Design review of the part built by this model. Coordinates are the model's own, in mm. A direction names the side the tool comes from. Round coordinates to 2 decimals unless told otherwise and drop trailing zeros. Loops run counter-clockwise (first coordinate to the right, second up) from the corner with the lowest first, then second, coordinate; pieces in that order, holes last. Notation, with made-up numbers: M 3,27 L 11,27 A12 ccw 11,34 Z; hole C -32.5,89.5 d10. An arc over 180 degrees is marked long. One line per item, written item: value. Start each with the question number.
Item 1: For faces 1 (the flat face through (1, -38.1, 452)), 2 (the flat face through (1, 38.1, 452)), 3 (the cylindrical face through (-4.96, 37.776, 320.08)), list the 3-axis set-ups (+Z, -Z, +X, -X, +Y, -Y) from which the entire face can be reached by the end or side of a thin tool; tool diameter is ignored.
Item 2: We need section D-D (z = 151). Write out the cut boundary in (x, y), then the cut area to 3 significant figures.
Item 3: We need section C-C (x = 14). Write out the cut boundary in (y, z), then the cut area to 3 significant figures.
Item 4: For line 1 along Y through (x, z) = (-44.5, 465); line 2 along Z through (x, y) = (40, 20.5); line 3 along Z through (x, y) = (-56.5, 7.5), list the stretches that pass through material, from the lowest coordinate up.
Item 5: We need section A-A (x = 43.5). Write out the cut boundary in (y, z), then the cut area to 3 significant figures.
Item 6: We need section B-B (y = 0). Write out the cut boundary in (x, z).
Item 7: Clearance check with flat-ended pins moving along their axes: pin 1 (2 mm diameter, centred on y = 3.5, z = 299, fed in from -X); pin 2 (6 mm diameter, centred on x = -10, y = -19, fed in from +Z); pin 3 (12 mm diameter, centred on y = 36.5, z = 132.5, fed in from -X). State where each tip first meets the part, or that it passes through.
Item 8: Mouldability with a two-part tool opening along Z and no side actions: class faces 4 (the flat face through (-1, 1, 0)), 5 (the flat face through (27.3, -27.3, 254)), 6 (the cylindrical face through (-13.77, -61.99, 125.22)) as released by +Z, released by -Z, zero draft, split by the parting line, or undercut.
from build123d import *

# Parameters (mm, degrees)
F0_R     = 63.5
F1_DEPTH = 254
F3_R     = 38.1
F2_DEPTH = 152.4
F4_W     = 76.2
F4_H     = 73.906902


with BuildPart() as f1:
    # F0 (on Top) → F1 (new body)
    with BuildSketch(Plane.XY):
        Circle(F0_R)
    extrude(amount=F1_DEPTH)

    # F3 (on face) → F2 (join)
    with BuildSketch(Plane.XY.offset(254)):
        Circle(F3_R)
    extrude(amount=F2_DEPTH)

    # F4 (on Right) → F5 (revolve)
    with BuildSketch(Plane.YZ):
        with Locations((0, 414.412725)):
            Rectangle(F4_W, F4_H)
    revolve(axis=Axis((0, 0, 451.366176), (0, -1, 0)))


solid = f1.part
A:
1. face 1: +Z, +X, -X, -Y
1. face 2: +Z, +X, -X, +Y
1. face 3: none
2. outline: C 0,0 d127
2. area: 12,700 mm2
3. outline: M -61.94,0 L 61.94,0 L 61.94,254 L 35.43,254 L 35.43,378.8 L 38.1,378.8 L 38.1,523.93 L -38.1,523.93 L -38.1,378.8 L -35.43,378.8 L -35.43,254 L -61.94,254 Z
3. area: 51,400 mm2
4. line 1: -38.1 to 38.1
4. line 2: 0 to 254, 389.22 to 513.51
4. line 3: 0 to 254, 403.72 to 499.01
5. outline: M -46.26,0 L 46.26,0 L 46.26,254 L -46.26,254 Z; M -38.1,391.62 L 38.1,391.62 L 38.1,511.12 L -38.1,511.12 Z
5. area: 32,600 mm2
6. outline: M -63.5,0 L 63.5,0 L 63.5,254 L 38.1,254 L 38.1,388.04 A73.91 ccw long -38.1,388.04 L -38.1,254 L -63.5,254 Z
7. pin 1: x = -38.02
7. pin 2: z = 524.94
7. pin 3: x = -55.7
8. face 4: released by -Z
8. face 5: undercut
8. face 6: zero draft
